Model file for the job. Use its own axes, mm. Face numbers are marked on the shaded views. A direction names the side the tool comes from. Coordinates: 2 decimals unless noted, no trailing zeros. Loops run counter-clockwise (first coordinate to the right, second up) from the corner with the lowest first, then second, coordinate; pieces in that order, holes last.
from build123d import *

# Parameters (mm, degrees)
F0_R      = 19.05
F1_DEPTH  = 20.955
F3_DEPTH  = 25.4
F5_DEPTH  = 25.4
F6_R      = 4.572
F7_DEPTH  = 17.145
F9_D      = 3.4544
F9_DEPTH  = 10.81405
F9_TIP    = 1.0378064612
F11_R     = 6.35
F12_DEPTH = 1.5875
F14_DEPTH = 3.302


# Not quite as in the source:
# - a feature names something its author has since deleted; it is built from what else it names


with BuildPart() as f1:
    # F0 (on Top) → F1 (new body)
    with BuildSketch(Plane.XY):
        Circle(F0_R)
    extrude(amount=-F1_DEPTH)

    # F2 (on Right) → F3 (cut, symmetric)
    with BuildSketch(Plane.YZ):
        Polygon((-10.3632, -0.7493), (-10.3632, 0), (-19.05, 0), (-19.05, -5.08), (-6.0325, -5.08), align=None)
        Polygon((10.3632, -0.7493), (6.0325, -5.08), (19.05, -5.08), (19.05, 0), (10.3632, 0), align=None)
    extrude(amount=F3_DEPTH, both=True, mode=Mode.SUBTRACT)

    # F4 (on Right) → F5 (cut, symmetric)
    with BuildSketch(Plane.YZ):
        with BuildLine():
            Line((-19.05, -20.955), (-9.525, -20.955))
            Line((-9.525, -20.955), (-9.525, -12.192))
            ThreePointArc((-9.525, -12.192), (-10.4549359697, -9.9469359697), (-12.7, -9.017))
            Line((-12.7, -9.017), (-19.05, -9.017))
            Line((-19.05, -9.017), (-19.05, -20.955))
        make_face()
        with BuildLine():
            Line((19.05, -9.017), (12.7, -9.017))
            ThreePointArc((12.7, -9.017), (10.4549359697, -9.9469359697), (9.525, -12.192))
            Line((9.525, -12.192), (9.525, -20.955))
            Line((9.525, -20.955), (19.05, -20.955))
            Line((19.05, -20.955), (19.05, -9.017))
        make_face()
    extrude(amount=F5_DEPTH, both=True, mode=Mode.SUBTRACT)

    # F6 (on face) → F7 (cut)
    with BuildSketch(Plane(origin=(0, 0, -20.955), x_dir=(1, 0, 0), z_dir=(0, 0, -1))):
        Circle(F6_R)
        with Locations((-11.684, 0)):
            Circle(F6_R)
    extrude(amount=-F7_DEPTH, mode=Mode.SUBTRACT)

    # F9
    with Locations(Plane(origin=(0, 9.525, 0), x_dir=(-1, 0, 0), z_dir=(0, 1, 0))):
        with Locations((0, -14.2748), (11.684, -14.2748)):
            Hole(F9_D / 2, depth=F9_DEPTH)
            with Locations((0, 0, -(F9_DEPTH + F9_TIP / 2))):  # 118° drill point
                Cone(0, F9_D / 2, F9_TIP, mode=Mode.SUBTRACT)

    # F11 (on offset) → F12 (cut)
    with BuildSketch(Plane.YZ.offset(19.05)):
        with Locations((0, 3.81)):
            Circle(F11_R)
    extrude(amount=-F12_DEPTH, mode=Mode.SUBTRACT)

    # F13 (on face) → F14 (cut)
    with BuildSketch(Plane.XY):
        with BuildLine():
            Line((5.5499, 4.9276), (2.3241, 4.9276))
            ThreePointArc((2.3241, 4.9276), (1.2015679849, 4.4626320151), (0.7366, 3.3401))
            Line((0.7366, 3.3401), (0.7366, -3.3401))
            ThreePointArc((0.7366, -3.3401), (1.2015679849, -4.4626320151), (2.3241, -4.9276))
            Line((2.3241, -4.9276), (5.5499, -4.9276))
            ThreePointArc((5.5499, -4.9276), (6.6724320151, -4.4626320151), (7.1374, -3.3401))
            Line((7.1374, -3.3401), (7.1374, 3.3401))
            ThreePointArc((7.1374, 3.3401), (6.6724320151, 4.4626320151), (5.5499, 4.9276))
        make_face()
    extrude(amount=-F14_DEPTH, mode=Mode.SUBTRACT)


solid = f1.part
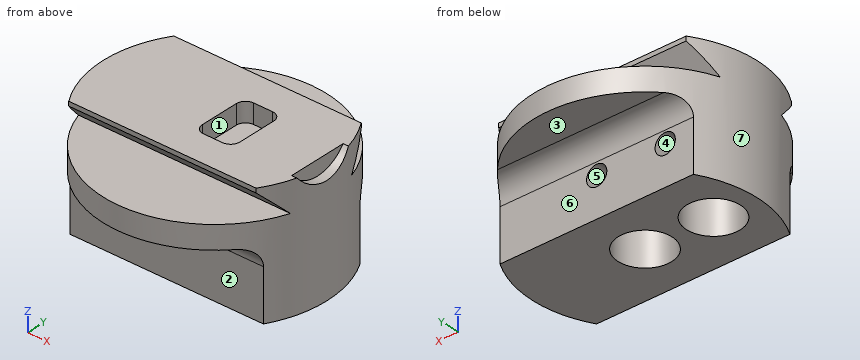
Q1. Slice it at D-D (z = -18.5). List the corners of the cut face in (x, y) (3 decimals).
Answers:
outline: (-16.498, -9.525) - (16.498, -9.525) arc R19.05 ccw to (16.498, 9.525) - (-16.498, 9.525) arc R19.05 ccw to start; hole circle Ø9.144 at (-11.684, 0); hole circle Ø9.144 at (0, 0)
Q2. Slice it at C-C (y = 9). List the corners of the cut face in (x, z) (1 decimal).
Answers:
outline: (-16.8, -21) - (16.8, -21) - (16.8, -5.1) - (-16.8, -5.1) - close; (-16.8, -2.1) - (16.8, -2.1) - (16.8, 0) - (-16.8, 0) - close; hole circle Ø3.5 at (-11.7, -14.3); hole circle Ø3.5 at (0, -14.3)
Q3. Flat gauge pins, fed straight in: P1, Ø8, axis at x = -13, y = -8, coming from the +Z side; P2, Ø2, axis at y = -1, z = -1.5, coming from the +X side; P3, Ø3.5, axis at x = 4, z = -1.5, coming from the -Y side; P4, Ø2, axis at x = -12.5, z = -18.5, coming from the +Y side (3 decimals). Where does each tip first touch, or does it go through?
Answers:
P1: stops at z = 0
P2: stops at x = 19.03
P3: stops at y = -10.36
P4: stops at y = 9.525
Q4. Which spindle directions (+Z, -Z, +X, -X, +Y, -Y) get a long thin tool onto all of the face, cutting with end or side? Do the marked faces 1, 2, 3 and 4. Say none if no direction does.
Answers:
face 1: +Z
face 2: -Z, +X, -X, -Y
face 3: -Z, +X, -X, +Y
face 4: +Y
Q5. Mould opens along X. For the marked faces 5, 6 and 7 say: +X half, -X half, draft (parallel to the pull), parting line (faces both ways), or undercut.
Answers:
face 5: undercut
face 6: draft
face 7: parting line
Q6. Drill centre lines: line 1 (X direction, y = 0, z = -8); line 2 (Z direction, x = 0, y = 8.2) (1 decimal); line 3 (X direction, y = -4, z = -12.25). Where is each one in solid material? Low to high.
Answers:
line 1: x = -19.05 to -16.26, -7.11 to -4.57, 4.57 to 19.05
line 2: z = -21 to -16, -12.5 to -5.1, -2.9 to 0
line 3: x = -18.63 to -13.9, -9.47 to -2.21, 2.21 to 18.63
